from build123d import *

# Parameters (mm, degrees)
EXTRUDE_1_DEPTH = 406.4


with BuildPart() as part:
    # 草图1 → 凸台-拉伸1 (new body)
    with BuildSketch(Plane.XY):
        with BuildLine():
            Line((0, 0), (35.98, 0))
            ThreePointArc((35.98, 0), (37.883814298, 0.788585702), (38.6724, 2.6924))
            Line((38.6724, 2.6924), (38.6724, 36.5252))
            ThreePointArc((38.6724, 36.5252), (33.8972, 41.3004), (29.122, 36.5252))
            ThreePointArc((29.122, 36.5252), (30.4682, 35.179), (31.8144, 36.5252))
            ThreePointArc((31.8144, 36.5252), (33.8972, 38.608), (35.98, 36.5252))
            Line((35.98, 36.5252), (35.98, 2.6924))
            Line((35.98, 2.6924), (0, 2.6924))
            Line((0, 2.6924), (0, 36.5252))
            ThreePointArc((0, 36.5252), (2.0828, 38.608), (4.1656, 36.5252))
            ThreePointArc((4.1656, 36.5252), (5.5118, 35.179), (6.858, 36.5252))
            ThreePointArc((6.858, 36.5252), (2.0828, 41.3004), (-2.6924, 36.5252))
            Line((-2.6924, 36.5252), (-2.6924, 2.6924))
            ThreePointArc((-2.6924, 2.6924), (-1.903814298, 0.788585702), (0, 0))
        make_face()
    extrude(amount=EXTRUDE_1_DEPTH)


solid = part.part
Read the model definition and answer for the solid it produces. Units are mm, in the model's axes. A direction names the side the tool comes from. Round coordinates to 2 decimals unless told otherwise and drop trailing zeros. Loops run counter-clockwise (first coordinate to the right, second up) from the corner with the lowest first, then second, coordinate; pieces in that order, holes last.
Q1. Each of these flat-tipped pins is pushed along its axis until it touches: pin 1 (12 mm diameter, centred on x = 21, y = 36.5, fed in from -Z); pin 2 (1.5 mm diameter, centred on x = 3.5, z = 116.5, fed in from +Y); pin 3 (2 mm diameter, centred on x = 23, z = 213, fed in from +Y). Where does it stop, or does it pass through?
Q2. Determine the mould class of faces 1 (the face through (38.672, 19, 200)), 2 (the face through (0, 19, 200)), 3 (the face through (18, 0, 200)) for opening direction X: released by +X, released by -X, zero draft, split by the parting line, or undercut.
Q3. Section C-C on x = 21 is taken. Write down the section's boundary in (y, z), and give its area (3 significant figures).
Q4. Section A-A on y = 31 is taken. Write down the section's boundary in (x, z), and give its area (3 significant figures).
Q5. Consider probe 1 along X at (y, z) = (36.5, 144); probe 2 along X at (y, z) = (11.5, 307); probe 3 along X at (y, z) = (37, 288). Determine where each line is inside the solid, lowest interval first.
Q6. Which of the six approach directions +Z, -Z, +X, -X, +Y, -Y give full straight-line access (tool end or side, diameter ignored) to faces 4 (the face through (18, 2.692, 200)), 5 (the face through (18, 2, 0))?
Output:
1. pin 1: passes through
1. pin 2: stops at y = 41.25
1. pin 3: stops at y = 2.69
2. face 1: released by +X
2. face 2: undercut
2. face 3: zero draft
3. outline: (0, 0) - (2.69, 0) - (2.69, 406.4) - (0, 406.4) - close
3. area: 1,090 mm2
4. outline: (-2.69, 0) - (0, 0) - (0, 406.4) - (-2.69, 406.4) - close; (35.98, 0) - (38.67, 0) - (38.67, 406.4) - (35.98, 406.4) - close
4. area: 2,190 mm2
5. probe 1: x = -2.69 to 0, 4.17 to 6.86, 29.12 to 31.81, 35.98 to 38.67
5. probe 2: x = -2.69 to 0, 35.98 to 38.67
5. probe 3: x = -2.67 to 0.05, 4.11 to 6.83, 29.15 to 31.87, 35.93 to 38.65
6. face 4: +Z, -Z
6. face 5: -Z, +X, -X, +Y, -Y
